Source: CAD feature listing. Evaluate the final solid. Frame: model axes, mm. A direction names the side the tool comes from. Give positions to 0.01 mm unless a question says otherwise; leave off trailing zeros. Order: outer loops, then holes, each group sorted by start corner. A loop starts at its lowest first (then second) coordinate and runs counter-clockwise, first axis right, second up.
from build123d import *

# Parameters (mm, degrees)
SKETCH1_R           = 100
BOSS_EXTRUDE1_DEPTH = 10
SKETCH2_R           = 25
BOSS_EXTRUDE2_DEPTH = 25
SKETCH3_W           = 15
SKETCH3_H           = 80
BOSS_EXTRUDE3_DEPTH = 70
CUT_EXTRUDE1_DEPTH  = 40
SKETCH7_W           = 40.381813508
SKETCH7_H           = 20
CUT_EXTRUDE2_DEPTH  = 208.25889607


with BuildPart() as part:
    # Sketch1 → Boss-Extrude1 (new body)
    with BuildSketch(Plane.XY):
        Circle(SKETCH1_R)
    extrude(amount=-BOSS_EXTRUDE1_DEPTH)

    # Sketch2 → Boss-Extrude2 (add)
    with BuildSketch(Plane(origin=(0, 0, -10), x_dir=(-1, 0, 0), z_dir=(0, 0, -1))):
        Circle(SKETCH2_R)
    extrude(amount=BOSS_EXTRUDE2_DEPTH)

    # Sketch3 → Boss-Extrude3 (add)
    with BuildSketch(Plane.XY):
        with Locations((-60, 0)):
            Rectangle(SKETCH3_W, SKETCH3_H)
    boss_extrude3 = extrude(amount=BOSS_EXTRUDE3_DEPTH)

    # Sketch5 → Cut-Extrude1 (cut)
    with BuildSketch(Plane.ZY.offset(67.5)):
        with BuildLine():
            Line((70, 0), (70, 40))
            Line((70, 40), (0, 40))
            Line((0, 40), (0, 13.288234805))
            Line((0, 13.288234805), (23.824003784, 13.288234805))
            ThreePointArc((23.824003784, 13.288234805), (51.913757827, 24.024986008), (70, 0))
        make_face()
        with BuildLine():
            Line((70, -40), (70, 0))
            ThreePointArc((70, 0), (51.913757827, -24.024986008), (23.824003784, -13.288234805))
            Line((23.824003784, -13.288234805), (0, -13.288234805))
            Line((0, -13.288234805), (0, -40))
            Line((0, -40), (70, -40))
        make_face()
    cut_extrude1 = extrude(amount=-CUT_EXTRUDE1_DEPTH, mode=Mode.SUBTRACT)

    # Mirror2: Boss-Extrude3, Cut-Extrude1 across plane
    add(boss_extrude3.mirror(Plane(origin=(0, 0, 0), x_dir=(0, 0, 1), z_dir=(1, 0, 0))))
    add(cut_extrude1.mirror(Plane(origin=(0, 0, 0), x_dir=(0, 0, 1), z_dir=(1, 0, 0))), mode=Mode.SUBTRACT)

    # Sketch7 → Cut-Extrude2 (cut, through all)
    with BuildSketch(Plane.ZY.offset(67.5)):
        with Locations((45, 0)):
            Rectangle(SKETCH7_W, SKETCH7_H)
    extrude(amount=-CUT_EXTRUDE2_DEPTH, mode=Mode.SUBTRACT)


solid = part.part
1) Section query B-B on x = 0. Output: boundary loops of the cut face in (y, z), and give its area (3 significant figures).
Checks:
outline: (-100, -10) - (-25, -10) - (-25, -35) - (25, -35) - (25, -10) - (100, -10) - (100, 0) - (-100, 0) - close
area: 3,250 mm2
2) Reachability of faces 5 (the face through (60, -10, 45)), 6 (the face through (-23.846, 7.509, -22.325)), 7 (the face through (-67.5, 11, 35)), 8 (the face through (-60, 13.288, 12)) from +Z, -Z, +X, -X, +Y, -Y: full face, straight path, thin tool, end or side. Return the list, or none.
Checks:
face 5: +X, -X
face 6: -Z
face 7: +Z, -X, +Y, -Y
face 8: +X, -X, +Y
3) Ray query, L1, parallel to X at y = -18, z = 34; L2, parallel to Z at x = 14, y = 35.5; L3, parallel to Z at x = -15.5, y = -13.5. Return the intervals inside material, ascending.
Checks:
L1: x = -67.5 to -52.5, 52.5 to 67.5
L2: z = -10 to 0
L3: z = -35 to 0
4) Pull-direction query (Y, two-part tool) for faces 1 (the face through (60, 0, 24.809)), 2 (the face through (-60, -10, 45)), 3 (the face through (60, 13.288, 12)), 4 (the face through (52.5, -11, 35)); classes: +Y half, -Y half, draft (parallel to the pull), parting line (faces both ways), or undercut.
Checks:
face 1: undercut
face 2: undercut
face 3: +Y half
face 4: draft
5) Section query A-A on z = 35. Output: boundary loops of the cut face in (x, y), and give its area (3 significant figures).
Checks:
outline: (-67.5, -22.91) - (-52.5, -22.91) - (-52.5, -10) - (-67.5, -10) - close; (-67.5, 10) - (-52.5, 10) - (-52.5, 22.91) - (-67.5, 22.91) - close; (52.5, -22.91) - (67.5, -22.91) - (67.5, -10) - (52.5, -10) - close; (52.5, 10) - (67.5, 10) - (67.5, 22.91) - (52.5, 22.91) - close
area: 775 mm2
6) Section query C-C on z = -14. Output: boundary loops of the cut face in (x, y).
Checks:
outline: circle Ø50 at (0, 0)
7) Section query D-D on z = 49.5. Output: boundary loops of the cut face in (x, y).
Checks:
outline: (-67.5, -24.59) - (-52.5, -24.59) - (-52.5, -10) - (-67.5, -10) - close; (-67.5, 10) - (-52.5, 10) - (-52.5, 24.59) - (-67.5, 24.59) - close; (52.5, -24.59) - (67.5, -24.59) - (67.5, -10) - (52.5, -10) - close; (52.5, 10) - (67.5, 10) - (67.5, 24.59) - (52.5, 24.59) - close
8) First-contact query: pin 1 Ø4.5 at (x, z) = (-63.5, 52.5) entering from +Y; pin 2 Ø7.5 at (x, z) = (-63, 7.5) entering from -Y; pin 3 Ø15 at (y, z) = (9.5, 21) entering from +X; pin 4 Ø8 at (y, z) = (-80, -16) entering from -X. Flat tips, straight axial feed; report the tip coordinate or a pass-through.
Checks:
pin 1: stops at y = 24.44
pin 2: stops at y = -13.29
pin 3: stops at x = 67.5
pin 4: passes through
